Design review of the part built by this model. Coordinates are the model's own, in mm. A direction names the side the tool comes from. Round coordinates to 2 decimals unless told otherwise and drop trailing zeros. Write each loop counter-clockwise with the first axis right and the second up, starting at its lowest first coordinate (ties: lowest second). Pieces come first, ordered by that corner, then holes. Notation, with made-up numbers: (-24.75, 68) - (31.25, 68) arc R36 ccw to (31.25, 106) - close; hole circle Ø2 at (5.25, 66). An arc over 180 degrees is marked (long way). Use one line per item in the form item = value.
```python
from build123d import *

# Parameters (mm, degrees)
SKETCH1_R            = 12.5
BOSS_EXTRUDE1_DEPTH  = 50
SKETCH3_R            = 15
BOSS_EXTRUDE2_DEPTH  = 15
SKETCH4_R            = 22.5
BOSS_EXTRUDE3_DEPTH  = 23
SKETCH5_R            = 22.5
BOSS_EXTRUDE5_DEPTH  = 18.56
SKETCH6_R            = 22.5
BOSS_EXTRUDE6_DEPTH  = 18.56
SKETCH7_R            = 25.5
BOSS_EXTRUDE7_DEPTH  = 2
SKETCH9_R            = 22.5
BOSS_EXTRUDE8_DEPTH  = 30
SKETCH11_R           = 25.5
BOSS_EXTRUDE9_DEPTH  = 2
BOSS_EXTRUDE10_DEPTH = 18.56
SKETCH13_R           = 22.5
BOSS_EXTRUDE11_DEPTH = 23
SKETCH14_R           = 15
BOSS_EXTRUDE12_DEPTH = 15
SKETCH15_R           = 12.5
BOSS_EXTRUDE13_DEPTH = 50


with BuildPart() as part:
    # Sketch1 → Boss-Extrude1 (new body)
    with BuildSketch(Plane.XY):
        Circle(SKETCH1_R)
    extrude(amount=-BOSS_EXTRUDE1_DEPTH)

    # Sketch3 → Boss-Extrude2 (add)
    with BuildSketch(Plane(origin=(0, 0, -50), x_dir=(-1, 0, 0), z_dir=(0, 0, -1))):
        Circle(SKETCH3_R)
    extrude(amount=BOSS_EXTRUDE2_DEPTH)

    # Sketch4 → Boss-Extrude3 (add)
    with BuildSketch(Plane(origin=(0, 0, -65), x_dir=(-1, 0, 0), z_dir=(0, 0, -1))):
        Circle(SKETCH4_R)
    extrude(amount=BOSS_EXTRUDE3_DEPTH)



with BuildPart() as body_2:
    # Sketch5 → Boss-Extrude5 (new body)
    with BuildSketch(Plane(origin=(0, 0, -88), x_dir=(-1, 0, 0), z_dir=(0, 0, -1))):
        with BuildLine():
            ThreePointArc((30.5, 40), (0, 70.5), (-30.5, 40))
            Line((-30.5, 40), (-30.5, 20))
            Line((-30.5, 20), (-59.999999922, -0.003051235))
            ThreePointArc((-59.999999922, -0.003051235), (0.001525617, -59.999999981), (60, 0))
            Line((60, 0), (30.5, 20))
            Line((30.5, 20), (30.5, 40))
        make_face()
        Circle(SKETCH5_R, mode=Mode.SUBTRACT)
    extrude(amount=BOSS_EXTRUDE5_DEPTH)


with BuildPart() as part_1:
    add(part.part)

    add(body_2.part)  # Boss-Extrude6 merges body 2
    # Sketch6 → Boss-Extrude6 (add)
    with BuildSketch(Plane(origin=(0, 0, -106.56), x_dir=(-1, 0, 0), z_dir=(0, 0, -1))):
        Circle(SKETCH6_R)
    extrude(amount=-BOSS_EXTRUDE6_DEPTH)

    # Sketch7 → Boss-Extrude7 (add)
    with BuildSketch(Plane(origin=(0, 0, -106.56), x_dir=(-1, 0, 0), z_dir=(0, 0, -1))):
        with Locations((0, 40)):
            Circle(SKETCH7_R)
    extrude(amount=BOSS_EXTRUDE7_DEPTH)

    # Sketch9 → Boss-Extrude8 (add)
    with BuildSketch(Plane(origin=(0, 0, -108.56), x_dir=(-1, 0, 0), z_dir=(0, 0, -1))):
        with Locations((0, 40)):
            Circle(SKETCH9_R)
    extrude(amount=BOSS_EXTRUDE8_DEPTH)

    # Sketch11 → Boss-Extrude9 (add)
    with BuildSketch(Plane(origin=(0, 0, -138.56), x_dir=(-1, 0, 0), z_dir=(0, 0, -1))):
        with Locations((0, 40)):
            Circle(SKETCH11_R)
    extrude(amount=BOSS_EXTRUDE9_DEPTH)

    # Sketch12 → Boss-Extrude10 (add)
    with BuildSketch(Plane(origin=(0, 0, -140.56), x_dir=(-1, 0, 0), z_dir=(0, 0, -1))):
        with BuildLine():
            Line((-30.5, 40), (-30.5, 20))
            Line((-30.5, 20), (-60, 0))
            ThreePointArc((-60, 0), (0, -60), (60, 0))
            Line((60, 0), (30.5, 20))
            Line((30.5, 20), (30.5, 40))
            ThreePointArc((30.5, 40), (0, 70.5), (-30.5, 40))
        make_face()
    extrude(amount=BOSS_EXTRUDE10_DEPTH)

    # Sketch13 → Boss-Extrude11 (add)
    with BuildSketch(Plane(origin=(0, 0, -159.12), x_dir=(-1, 0, 0), z_dir=(0, 0, -1))):
        Circle(SKETCH13_R)
    extrude(amount=BOSS_EXTRUDE11_DEPTH)

    # Sketch14 → Boss-Extrude12 (add)
    with BuildSketch(Plane(origin=(0, 0, -182.12), x_dir=(-1, 0, 0), z_dir=(0, 0, -1))):
        Circle(SKETCH14_R)
    extrude(amount=BOSS_EXTRUDE12_DEPTH)

    # Sketch15 → Boss-Extrude13 (add)
    with BuildSketch(Plane(origin=(0, 0, -197.12), x_dir=(-1, 0, 0), z_dir=(0, 0, -1))):
        Circle(SKETCH15_R)
    extrude(amount=BOSS_EXTRUDE13_DEPTH)


solid = part_1.part
```
Q1. We need section B-B on z = -155. Write out the cut boundary in (x, y), then the cut area to 3 significant figures.
Calculated:
outline = (-60, 0) arc R60 ccw to (60, 0) - (30.5, 20) - (30.5, 40) arc R30.5 ccw to (-30.5, 40) - (-30.5, 20) - close
area = 10,100 mm2
Q2. Draft analysis for pull direction Z (two halves, no side actions). For faces 1 (the flat face through (45.04, 10.14, -97.15)), 2 (the cylindrical face through (-13.71, 61.5, -139.55)), 3 (the flat face through (0, 0, 0)), state which applies: released by +Z, released by -Z, zero draft, split by the parting line, or undercut.
Calculated:
face_1 = zero draft
face_2 = undercut
face_3 = released by +Z
Q3. We need section A-A on y = -39. Write out the cut boundary in (x, z).
Calculated:
outline = (-45.6, -159.12) - (45.6, -159.12) - (45.6, -140.56) - (-45.6, -140.56) - close; (-45.6, -106.56) - (45.6, -106.56) - (45.6, -88) - (-45.6, -88) - close
Q4. To check wall thickness, follow line 1 along Z through (x, y) = (18.5, 62.5); line 2 along Z through (x, y) = (9, 39); line 3 along Y through (x, z) = (-49, -148.5). State the ranges of each line that lie inside material, in increasing order. Write a range as from..to.
Calculated:
line_1 = -159.12..-140.56, -106.56..-88
line_2 = -159.12..-88
line_3 = -34.63..7.46
Q5. Machinability: for faces 4 (the cylindrical face through (14.985, 0.66, -189.515)), 5 (the cylindrical face through (11.923, 3.755, -24.65)), 6 (the flat face through (30.5, 30, -150)), 7 (the cylindrical face through (-13.71, 61.5, -107.55)), which of the approach directions +Z, -Z, +X, -X, +Y, -Y give a long, thin tool a straight path to every point of the face, cutting with its end or side? Answer none if there is none.
Calculated:
face_4 = -Z
face_5 = +Z
face_6 = +Z, -Z, +X, +Y
face_7 = none
Q6. We need section C-C on x = -36. Write out the cut boundary in (y, z).
Calculated:
outline = (-48, -159.12) - (16.27, -159.12) - (16.27, -140.56) - (-48, -140.56) - close; (-48, -106.56) - (16.27, -106.56) - (16.27, -88) - (-48, -88) - close
Q7. For P1, Ø4, axis at x = -4, z = -75, coming from the +Y side; P2, Ø1.5, axis at x = -15, z = -109.5, coming from the -Y side; P3, Ø20.5, axis at y = 31.5, z = -99.5, coming from the -X side, all flat-tipped, find the tip position at first contact; note any pin that passes through.
Calculated:
P1 = 22.41
P2 = 22.59
P3 = -30.5
